Read the model definition and answer for the solid it produces. Units are mm, in the model's axes. Coordinates: 2 decimals unless noted, no trailing zeros. Loops run counter-clockwise (first coordinate to the right, second up) from the corner with the lowest first, then second, coordinate; pieces in that order, holes last.
Q1. Straight lines are drawn through the part: line 1 (Y direction, x = 71.5, z = 2.5); line 2 (Y direction, x = 250, z = 1.6); line 3 (Y direction, x = 172.5, z = 2.05). For each, find the intervals that lie inside material, in ascending order.
Q2. Section B-B (z = 0.8) is taken. Count the separate pieces of the cut face and the enclosed holes in it, then the cut area to 3 significant figures.
Q3. Section A-A (x = 194.5) is taken. Give the vertices of the cut face in (y, z).
Q4. Flat-ended cylindrical pins translate along their axes: P1, Ø1.5, axis at x = 276.5, z = 1.5, coming from the +Y side; P2, Ø0.9, axis at x = 60, z = 1, coming from the -Y side. Find the tip coordinate at first contact, or state that the pin passes through.
Autodesk Inventor part; units mm, degrees
ref_plane "YZ Plane" through (0, 0, 0) normal (1, 0, 0) x (0, 1, 0)
ref_plane "XZ Plane" through (0, 0, 0) normal (0, 1, 0) x (-1, 0, 0)
ref_plane "XY Plane" through (0, 0, 0) normal (0, 0, 1) x (1, 0, 0)
sketch "Sketch1" plane through (0, 0, 0) normal (0, 0, 1) x (1, 0, 0)
  line L0 (0, 0) -> (280, 0)
  line L1 (280, 0) -> (280, 16)
  line L2 (280, 16) -> (0, 16)
  line L3 (0, 16) -> (0, 0)
  line L4 (0, 0) -> (22.0483, 0)
  line L5 (10, 0) -> (29.5, 0)
  line L6 (29.5, 0) -> (29.5, -5)
  line L7 (29.5, -5) -> (10, -5)
  line L8 (10, -5) -> (10, 0)
  line L9 (8.4, 13.1) -> (11.6, 13.1)
  line L10 (11.6, 13.1) -> (11.6, 2.9)
  line L11 (11.6, 2.9) -> (8.4, 2.9)
  line L12 (8.4, 2.9) -> (8.4, 13.1)
  line L13 (8.4, 13.1) -> (11.6, 2.9) construction
  line L14 (11.6, 13.1) -> (8.4, 2.9) construction
  line L15 (268.4, 13.1) -> (271.6, 13.1)
  line L16 (271.6, 13.1) -> (271.6, 2.9)
  line L17 (271.6, 2.9) -> (268.4, 2.9)
  line L18 (268.4, 2.9) -> (268.4, 13.1)
  line L19 (268.4, 13.1) -> (271.6, 2.9) construction
  line L20 (271.6, 13.1) -> (268.4, 2.9) construction
  circle A0 centre (260, 11) radius 2.05
  circle A1 centre (250, 11) radius 2.05
  line L21 (48.4, 13.1) -> (51.6, 13.1)
  line L22 (51.6, 13.1) -> (51.6, 2.9)
  line L23 (51.6, 2.9) -> (48.4, 2.9)
  line L24 (48.4, 2.9) -> (48.4, 13.1)
  line L25 (48.4, 13.1) -> (51.6, 2.9) construction
  line L26 (51.6, 13.1) -> (48.4, 2.9) construction
  line L27 (88.4, 13.1) -> (91.6, 13.1)
  line L28 (91.6, 13.1) -> (91.6, 2.9)
  line L29 (91.6, 2.9) -> (88.4, 2.9)
  line L30 (88.4, 2.9) -> (88.4, 13.1)
  line L31 (88.4, 13.1) -> (91.6, 2.9) construction
  line L32 (91.6, 13.1) -> (88.4, 2.9) construction
  line L33 (128.4, 13.1) -> (131.6, 13.1)
  line L34 (131.6, 13.1) -> (131.6, 2.9)
  line L35 (131.6, 2.9) -> (128.4, 2.9)
  line L36 (128.4, 2.9) -> (128.4, 13.1)
  line L37 (128.4, 13.1) -> (131.6, 2.9) construction
  line L38 (131.6, 13.1) -> (128.4, 2.9) construction
  line L39 (168.4, 13.1) -> (171.6, 13.1)
  line L40 (171.6, 13.1) -> (171.6, 2.9)
  line L41 (171.6, 2.9) -> (168.4, 2.9)
  line L42 (168.4, 2.9) -> (168.4, 13.1)
  line L43 (168.4, 13.1) -> (171.6, 2.9) construction
  line L44 (171.6, 13.1) -> (168.4, 2.9) construction
  line L45 (188.4, 13.1) -> (191.6, 13.1)
  line L46 (191.6, 13.1) -> (191.6, 2.9)
  line L47 (191.6, 2.9) -> (188.4, 2.9)
  line L48 (188.4, 2.9) -> (188.4, 13.1)
  line L49 (188.4, 13.1) -> (191.6, 2.9) construction
  line L50 (191.6, 13.1) -> (188.4, 2.9) construction
  line L51 (31.6, 13.1) -> (31.6, 2.9)
  line L52 (28.4, 13.1) -> (31.6, 13.1)
  line L53 (28.4, 2.9) -> (28.4, 13.1)
  line L54 (31.6, 13.1) -> (28.4, 2.9) construction
  line L55 (31.6, 2.9) -> (28.4, 2.9)
  line L56 (28.4, 13.1) -> (31.6, 2.9) construction
  line L57 (71.6, 13.1) -> (71.6, 2.9)
  line L58 (68.4, 13.1) -> (71.6, 13.1)
  line L59 (68.4, 2.9) -> (68.4, 13.1)
  line L60 (71.6, 13.1) -> (68.4, 2.9) construction
  line L61 (71.6, 2.9) -> (68.4, 2.9)
  line L62 (68.4, 13.1) -> (71.6, 2.9) construction
  line L63 (41.6, 13.1) -> (41.6, 2.9)
  line L64 (38.4, 13.1) -> (41.6, 13.1)
  line L65 (38.4, 2.9) -> (38.4, 13.1)
  line L66 (41.6, 13.1) -> (38.4, 2.9) construction
  line L67 (41.6, 2.9) -> (38.4, 2.9)
  line L68 (38.4, 13.1) -> (41.6, 2.9) construction
  line L69 (61.6, 13.1) -> (61.6, 2.9)
  line L70 (58.4, 13.1) -> (61.6, 13.1)
  line L71 (58.4, 2.9) -> (58.4, 13.1)
  line L72 (61.6, 13.1) -> (58.4, 2.9) construction
  line L73 (61.6, 2.9) -> (58.4, 2.9)
  line L74 (58.4, 13.1) -> (61.6, 2.9) construction
  point P0 (10, 8)
  point P1 (0, 8)
  point P2 (270, 8)
  point P3 (50, 8)
  point P4 (90, 8)
  point P5 (130, 8)
  point P6 (170, 8)
  point P7 (190, 8)
  point P8 (30, 8)
  point P9 (70, 8)
  point P10 (40, 8)
  point P11 (60, 8)
  dimension "d2" = 19.5
  dimension "d3" = 5
  dimension "d4" = 10
  dimension "d5" = 16
  dimension "d8" = 280
  dimension "d10" = 10.2
  dimension "d11" = 3.2
  dimension "d12" = 10
  dimension "d13" = 10.2
  dimension "d14" = 3.2
  dimension "d15" = 10
  dimension "d16" = 4.1
  dimension "d18" = 4.1
  dimension "d20" = 10
  dimension "d21" = 20
  dimension "d23" = 5
  dimension "d26" = 10.2
  dimension "d27" = 3.2
  dimension "d28" = 10.2
  dimension "d29" = 3.2
  dimension "d30" = 10.2
  dimension "d31" = 3.2
  dimension "d32" = 10.2
  dimension "d33" = 3.2
  dimension "d34" = 10.2
  dimension "d35" = 3.2
  dimension "d36" = 40
  dimension "d37" = 40
  dimension "d38" = 40
  dimension "d39" = 40
  dimension "d40" = 20
  dimension "d41" = 10.2
  dimension "d42" = 3.2
  dimension "d43" = 20
  dimension "d54" = 10.2
  dimension "d55" = 3.2
  dimension "d56" = 10.2
  dimension "d57" = 3.2
  dimension "d58" = 10.2
  dimension "d59" = 3.2
  dimension "d60" = 10
  dimension "d61" = 10
  dimension "d62" = 10
extrude "Extrusion1" add sketch "Sketch1" along normal blind 3
sketch "Sketch2" plane through (0, 0, 3) normal (0, 0, 1) x (1, 0, 0)
  line L0 (0, 16) -> (0, 0)
  line L1 (0, 16) -> (0, 41)
  line L2 (280, 0) -> (280, 16)
  line L3 (280, 16) -> (280, 41)
  line L4 (280, 41) -> (0, 41)
  line L5 (280, 16) -> (0, 16)
  line L6 (50, 16) -> (50, 31)
  line L7 (50, 31) -> (210, 31)
  line L8 (210, 31) -> (210, 16)
  line L9 (40, 41) -> (36, 51)
  line L10 (36, 51) -> (42, 51)
  line L11 (42, 51) -> (46, 41)
  circle A0 centre (250, 31) radius 2.05
  circle A1 centre (260, 31) radius 2.05
  circle A2 centre (250, 21) radius 2.05
  circle A3 centre (260, 21) radius 2.05
  circle A4 centre (260, 11) radius 2.05
  line L12 (268.4, 33.1) -> (271.6, 33.1)
  line L13 (271.6, 33.1) -> (271.6, 22.9)
  line L14 (271.6, 22.9) -> (268.4, 22.9)
  line L15 (268.4, 22.9) -> (268.4, 33.1)
  line L16 (268.4, 33.1) -> (271.6, 22.9) construction
  line L17 (271.6, 33.1) -> (268.4, 22.9) construction
  line L18 (268.4, 13.1) -> (271.6, 13.1)
  line L19 (271.6, 13.1) -> (271.6, 2.9)
  line L20 (274.4, 33.1) -> (277.6, 33.1)
  line L21 (277.6, 33.1) -> (277.6, 22.9)
  line L22 (277.6, 22.9) -> (274.4, 22.9)
  line L23 (274.4, 22.9) -> (274.4, 33.1)
  line L24 (274.4, 33.1) -> (277.6, 22.9) construction
  line L25 (277.6, 33.1) -> (274.4, 22.9) construction
  point P0 (270, 28)
  point P1 (270, 13.1)
  point P2 (271.6, 8)
  point P3 (276, 28)
  dimension "d44" = 25
  dimension "d45" = 160
  dimension "d46" = 50
  dimension "d47" = 15
  dimension "d48" = 10
  dimension "d49" = 6
  dimension "d50" = 4
  dimension "d51" = 40
  dimension "d63" = 4.1
  dimension "d64" = 4.1
  dimension "d65" = 4.1
  dimension "d66" = 4.1
  dimension "d67" = 20
  dimension "d68" = 10
  dimension "d69" = 10
  dimension "d70" = 10
  dimension "d71" = 10.2
  dimension "d72" = 20
  dimension "d73" = 3.2
  dimension "d74" = 6
extrude "Extrusion2" add sketch "Sketch2" against normal blind 3 contours L1 L4 L3 L5 L8 L7 L6 | L9 L10 L11 L4
properties part number "Middle_bar"
Numbers:
1. line 1: y = 0 to 2.9, 13.1 to 16, 31 to 41
1. line 2: y = 0 to 8.95, 13.05 to 18.95, 23.05 to 28.95, 33.05 to 41
1. line 3: y = 0 to 16, 31 to 41
2. separate pieces: 1
2. enclosed holes: 20
2. area: 8,730 mm2
3. outline: (0, 0) - (16, 0) - (16, 3) - (0, 3) - close; (31, 0) - (41, 0) - (41, 3) - (31, 3) - close
4. P1: stops at y = 41
4. P2: stops at y = 0
